Geometry check sheet. Reference: the model listing, model coordinates, mm. Face numbers are marked on the shaded views. Round coordinates to 2 decimals unless told otherwise and drop trailing zeros. Write each loop counter-clockwise with the first axis right and the second up, starting at its lowest first coordinate (ties: lowest second). Pieces come first, ordered by that corner, then holes. Notation, with made-up numbers: (-16, 80) -> (-11, 80) arc R29 ccw to (-11, 106) -> close; hole circle Ø1 at (-39.5, -11.75). An arc over 180 degrees is marked (long way). One line per question, with ' | ' between items.
```python
from build123d import *

# Parameters (mm, degrees)
SKETCH_W      = 26
SKETCH_H      = 26
SKETCH_R      = 7.1
EXTRUDE_DEPTH = 2
FILLET_R      = 3


with BuildPart() as part:
    # Sketch → Extrude (new body)
    with BuildSketch(Plane.XY):
        Rectangle(SKETCH_W, SKETCH_H)
        Circle(SKETCH_R, mode=Mode.SUBTRACT)
    extrude(amount=EXTRUDE_DEPTH)

    # Fillet
    fillet_edges = [part.edges().sort_by_distance(p)[0] for p in [
        (-13, -13, 1),
        (13, -13, 1),
        (13, 13, 1),
        (-13, 13, 1),
    ]]
    fillet(fillet_edges, radius=FILLET_R)


solid = part.part
```
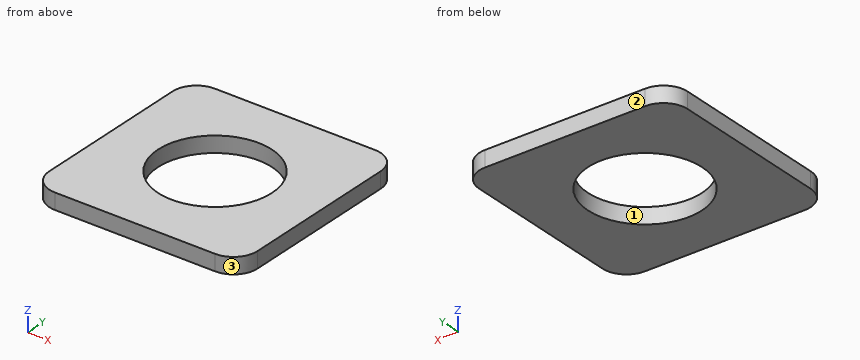
(1) Sectioned sample at B-B on z = 1.45. Record the cut outline in (x, y).
Resolved:
outline: (-13, -10) arc R3 ccw to (-10, -13) -> (10, -13) arc R3 ccw to (13, -10) -> (13, 10) arc R3 ccw to (10, 13) -> (-10, 13) arc R3 ccw to (-13, 10) -> close; hole circle Ø14.2 at (0, 0)
(2) Sectioned sample at A-A on y = 0. Record the cut outline in (x, z).
Resolved:
outline: (-13, 0) -> (-7.1, 0) -> (-7.1, 2) -> (-13, 2) -> close; (7.1, 0) -> (13, 0) -> (13, 2) -> (7.1, 2) -> close
(3) Draft check along Y on the marked faces 1, 2 and 3. Enter one of: +Y half, -Y half, draft (parallel to the pull), parting line (faces both ways), or undercut.
Resolved:
face 1: undercut | face 2: +Y half | face 3: -Y half
(4) Material ranges on line 1 (Y direction, x = 0, z = 0.55); line 2 (Y direction, x = -2.25, z = 1.6); line 3 (X direction, y = -5.5, z = 1.75), recorded low to high.
Resolved:
line 1: y = -13 to -7.1, 7.1 to 13 | line 2: y = -13 to -6.73, 6.73 to 13 | line 3: x = -13 to -4.49, 4.49 to 13
